Build history of the part. All positions in model axes, mm. Give positions to 0.01 mm unless a question says otherwise; leave off trailing zeros. Loops run counter-clockwise (first coordinate to the right, second up) from the corner with the lowest first, then second, coordinate; pieces in that order, holes last. Notation, with made-up numbers: (52, -3) -> (104, -3) arc R23 ccw to (104, 30) -> close; hole circle Ø8 at (-30.75, -35.5). An arc over 180 degrees is marked (long way). Answer as a JSON object with one key per item and string values. Group by question number.
Q1. Band-saw the part on C-C, the plane y = 1.75. Write the cut outline in (x, z).
Q2. Band-saw the part on D-D, the plane z = 0. Write the cut outline in (x, y).
Q3. Two-plate mould, pull along Z, no slides. Class faces 1 (the flat face through (-8, 4, -55)), 2 (the flat face through (53, 4, 7)), 3 (the cylindrical face through (-42.9, 3.9, -43.2)): pulls with the +Z half, pulls with the -Z half, needs draft (parallel to the pull), parting line crosses it, or undercut.
Q4. Drop a flat-ended pin along its axis: pin 1 (2.5 mm diameter, centred on x = 42, z = -42, fed in from -Y). Give the stop position or say it passes through.
Q5. Band-saw the part on B-B, the plane x = -42. Write the cut outline in (y, z).
Q6. Wall check: probe 1 along X at (y, z) = (5.25, 42); probe 2 along X at (y, z) = (0.5, -41.5); probe 3 along X at (y, z) = (6, 6). Give the ranges that are in metal, low to high. Write a range as from..to.
Q7. Band-saw the part on A-A, the plane z = 42. Write the cut outline in (x, y).
from build123d import *

# Parameters (mm, degrees)
SKETCH1_W           = 108
SKETCH1_H           = 110
SKETCH1_R           = 19.15
SKETCH1_R_2         = 1.5
BOSS_EXTRUDE1_DEPTH = 8
FILLET1_R           = 12


with BuildPart() as part:
    # Sketch1 → Boss-Extrude1 (new body)
    with BuildSketch(Plane(origin=(0, 0, 0), x_dir=(1, 0, 0), z_dir=(0, 1, 0))):
        with Locations((-1, 0)):
            Rectangle(SKETCH1_W, SKETCH1_H)
        with Locations(Location((0, 0, 0), (0, 0, 270))):
            Circle(SKETCH1_R, mode=Mode.SUBTRACT)
        with Locations(Location((-42, 42, 0), (0, 0, 270))):
            Circle(SKETCH1_R_2, mode=Mode.SUBTRACT)
        with Locations(Location((42, 42, 0), (0, 0, 270))):
            Circle(SKETCH1_R_2, mode=Mode.SUBTRACT)
        with Locations(Location((42, -42, 0), (0, 0, 270))):
            Circle(SKETCH1_R_2, mode=Mode.SUBTRACT)
        with Locations(Location((-42, -42, 0), (0, 0, 270))):
            Circle(SKETCH1_R_2, mode=Mode.SUBTRACT)
    extrude(amount=BOSS_EXTRUDE1_DEPTH)

    # Fillet1
    fillet1_edges = [part.edges().sort_by_distance(p)[0] for p in [
        (53, 4, -55),
    ]]
    fillet(fillet1_edges, radius=FILLET1_R)


solid = part.part
Worked answers:
{
 "1": {"outline": "(-55, -55) -> (41, -55) arc R12 ccw to (53, -43) -> (53, 55) -> (-55, 55) -> close; hole circle Ø3 at (-42, -42); hole circle Ø3 at (-42, 42); hole circle Ø38.3 at (0, 0); hole circle Ø3 at (42, -42); hole circle Ø3 at (42, 42)"},
 "2": {"outline": "(-55, 0) -> (-19.15, 0) -> (-19.15, 8) -> (-55, 8) -> close; (19.15, 0) -> (53, 0) -> (53, 8) -> (19.15, 8) -> close"},
 "3": {"face 1": "pulls with the -Z half", "face 2": "needs draft", "face 3": "undercut"},
 "4": {"pin 1": "through"},
 "5": {"outline": "(0, -55) -> (8, -55) -> (8, -43.5) -> (0, -43.5) -> close; (0, -40.5) -> (8, -40.5) -> (8, 40.5) -> (0, 40.5) -> close; (0, 43.5) -> (8, 43.5) -> (8, 55) -> (0, 55) -> close"},
 "6": {"probe 1": "-55..-43.5, -40.5..40.5, 43.5..53", "probe 2": "-55..-43.41, -40.59..40.59, 43.41..53", "probe 3": "-55..-18.19, 18.19..53"},
 "7": {"outline": "(-55, 0) -> (-43.5, 0) -> (-43.5, 8) -> (-55, 8) -> close; (-40.5, 0) -> (40.5, 0) -> (40.5, 8) -> (-40.5, 8) -> close; (43.5, 0) -> (53, 0) -> (53, 8) -> (43.5, 8) -> close"}
}
